from build123d import *

# Parameters (mm, degrees)
F0_W     = 406.4
F0_H     = 15.875
F1_DEPTH = 762
F4_W     = 19.05
F4_H     = 406.4
F5_DEPTH = 1219.2


with BuildPart() as f1:
    # F0 (on Right) → F1 (new body)
    with BuildSketch(Plane.YZ):
        with Locations((203.2, 7.9375)):
            Rectangle(F0_W, F0_H)
    extrude(amount=F1_DEPTH)

    # F2: F1 across plane


with BuildPart() as f1_1:
    add(f1.part)
    add(f1.part.mirror(Plane.YZ))

    # F4 (on face) → F5 (join)
    with BuildSketch(Plane(origin=(0, 0, 0), x_dir=(1, 0, 0), z_dir=(0, 0, -1))):
        with Locations((-208.782977, -203.2)):
            Rectangle(F4_W, F4_H)
    extrude(amount=-F5_DEPTH)


solid = f1_1.part
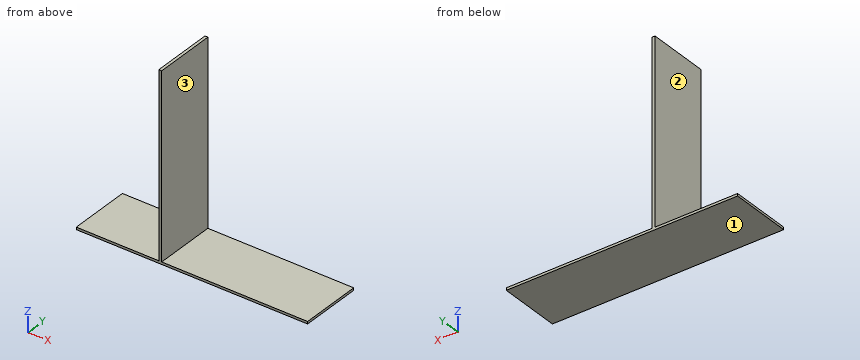
Can you work these out from the model? Positions are in its coordinate system, mm. Face numbers are marked on the shaded views. A direction names the side the tool comes from. Round coordinates to 2 decimals unless told otherwise and drop trailing zeros. Write each loop counter-clockwise with the first axis right and the second up, starting at its lowest first coordinate (ties: lowest second). Pieces come first, ordered by that corner, then holes. Notation, with made-up numbers: M 38.5,89 L 66.5,89 A28 ccw 66.5,116 Z; hole C 81.25,-17 d1. An arc over 180 degrees is marked long. Use a Markdown table: item, result.
Item 1: If I drill on line 1 along X through (y, z) = (19, 236.5); line 2 along Z through (x, y) = (-179.5, 55.5) (3 decimals), over which ranges is the centre line in solid material (lowest first)? Write a range as [from, to].
Found:
| item | result |
|---|---|
| line 1 | x = [-218.31, -199.26] |
| line 2 | z = [0, 15.875] |
Item 2: I want a section at A-A (y = 70). List the corners of the cut face in (x, z) for me (3 decimals), and give its area (3 significant figures).
Found:
| item | result |
|---|---|
| outline | M -762,0 L 762,0 L 762,15.875 L -199.258,15.875 L -199.258,1219.2 L -218.308,1219.2 L -218.308,15.875 L -762,15.875 Z |
| area | 47,100 mm2 |
Item 3: I want a section at B-B (z = 596). List the corners of the cut face in (x, y) for me, and give its area (3 significant figures).
Found:
| item | result |
|---|---|
| outline | M -218.31,0 L -199.26,0 L -199.26,406.4 L -218.31,406.4 Z |
| area | 7,740 mm2 |
Item 4: I want a section at C-C (x = 400). List the corners of the cut face in (y, z) for me (3 decimals).
Found:
| item | result |
|---|---|
| outline | M 0,0 L 406.4,0 L 406.4,15.875 L 0,15.875 Z |
Item 5: Which directions (+Z, -Z, +X, -X, +Y, -Y) give clear straight access to the entire face, cutting with the end or side of a thin tool? Please do the marked faces 1, 2 and 3.
Found:
| item | result |
|---|---|
| face 1 | -Z, +X, -X, +Y, -Y |
| face 2 | +Z, -X, +Y, -Y |
| face 3 | +Z, +X, +Y, -Y |
Item 6: For pin 1 Ø12 at (x, y) = (337, 264) entering from +Z (3 decimals); pin 2 Ø3 at (y, z) = (61, 982) entering from -X; pin 3 Ø3 at (y, z) = (350.5, 1023) entering from +X; pin 4 Ø1.5 at (x, y) = (-580, 52) entering from -Z, each with a flat end and sliding along its axis, tell me the tip position at first contact or that it passes through.
Found:
| item | result |
|---|---|
| pin 1 | stops at z = 15.875 |
| pin 2 | stops at x = -218.31 |
| pin 3 | stops at x = -199.26 |
| pin 4 | stops at z = 0 |
